Check sheet for the drawn part. Datum: minimum x, y, z corner. Units: mm. Round coordinates to 2 decimals unless told otherwise and drop trailing zeros. Loops run counter-clockwise (first coordinate to the right, second up) from the corner with the lowest first, then second, coordinate; pieces in that order, holes last. Notation, with made-up numbers: (26, -24) -> (42, -24) arc R18 cw to (42, -3) -> close; hole circle Ø2 at (82.5, 14). An arc over 180 degrees is marked (long way). Write item = value, one per line. Start each with the question number.
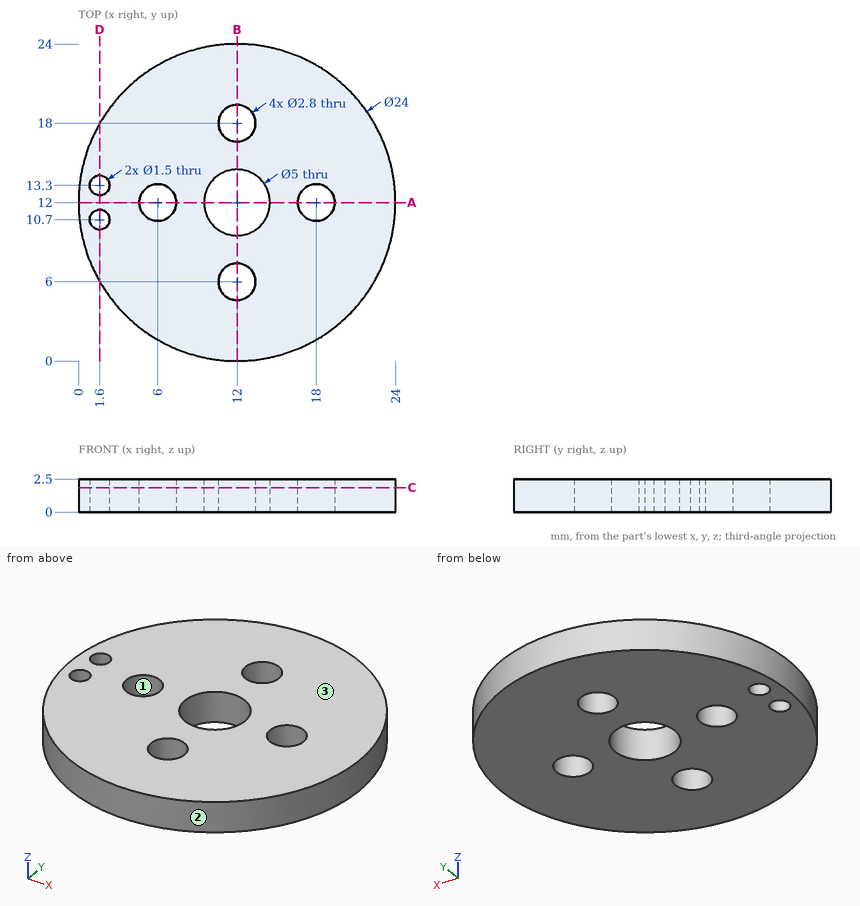
(1) Draft check along X on the marked faces 1, 2 and 3. Enter one of: +X half, -X half, draft (parallel to the pull), parting line (faces both ways), or undercut.
(2) Section check D-D on x = 1.6. Enter the section's corners in (y, z), then the cut area to 3 significant figures.
(3) Section check C-C on z = 1.85. Enter the section's corners in (x, y).
(4) Scan lines: line 1 (Y direction, x = 12, z = 1.1); line 2 (X direction, y = 11, z = 2.25); line 3 (Y direction, x = 1.6, z = 1.25). Record each from-to range of solid material in increasing order. Write a range as [from, to].
(5) Depth check by flat-ended pin: pin 1 Ø3.5 at (x, y) = (12, 6) entering from -Z; pin 2 Ø1 at (y, z) = (3.5, 0.5) entering from -X; pin 3 Ø4.5 at (x, y) = (12, 12) entering from -Z. Enter the tip coordinate at first touch or a pass-through.
(6) Section check A-A on y = 12. Enter the section's corners in (x, z), then the cut area to 3 significant figures.
Computed values:
q1.face_1 = undercut
q1.face_2 = parting line
q1.face_3 = draft
q2.outline = (6.01, 0) -> (9.95, 0) -> (9.95, 2.5) -> (6.01, 2.5) -> close; (11.45, 0) -> (12.55, 0) -> (12.55, 2.5) -> (11.45, 2.5) -> close; (14.05, 0) -> (17.99, 0) -> (17.99, 2.5) -> (14.05, 2.5) -> close
q2.area = 22.4 mm²
q3.outline = circle Ø24 at (12, 12); hole circle Ø1.5 at (1.6, 10.7); hole circle Ø1.5 at (1.6, 13.3); hole circle Ø2.8 at (6, 12); hole circle Ø5 at (12, 12); hole circle Ø2.8 at (12, 6); hole circle Ø2.8 at (12, 18); hole circle Ø2.8 at (18, 12)
q4.line_1 = [0, 4.6], [7.4, 9.5], [14.5, 16.6], [19.4, 24]
q4.line_2 = [0.04, 0.91], [2.29, 5.02], [6.98, 9.71], [14.29, 17.02], [18.98, 23.96]
q4.line_3 = [6.01, 9.95], [11.45, 12.55], [14.05, 17.99]
q5.pin_1 = 0
q5.pin_2 = 3.06
q5.pin_3 = through
q6.outline = (0, 0) -> (4.6, 0) -> (4.6, 2.5) -> (0, 2.5) -> close; (7.4, 0) -> (9.5, 0) -> (9.5, 2.5) -> (7.4, 2.5) -> close; (14.5, 0) -> (16.6, 0) -> (16.6, 2.5) -> (14.5, 2.5) -> close; (19.4, 0) -> (24, 0) -> (24, 2.5) -> (19.4, 2.5) -> close
q6.area = 33.5 mm²
